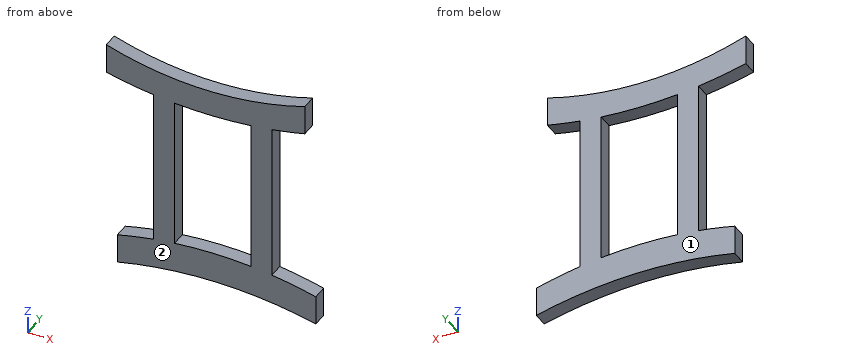
from build123d import *

# Parameters (mm, degrees)
F1_DEPTH = 6.604


with BuildPart() as f1:
    # F0 (on Front) → F1 (new body)
    with BuildSketch(Plane.XZ):
        with BuildLine():
            ThreePointArc((-43.79801, -38.727241), (-0.659432, -34.440726), (42.30799, -40.195004))
            Line((42.30799, -40.195004), (42.30799, -27.495004))
            ThreePointArc((42.30799, -27.495004), (32.83759, -25.203711), (23.254529, -23.442051))
            Line((23.254529, -23.442051), (23.254529, 44.543938))
            ThreePointArc((23.254529, 44.543938), (30.416051, 45.697065), (37.527271, 47.128027))
            Line((37.527271, 47.128027), (37.527271, 59.828027))
            ThreePointArc((37.527271, 59.828027), (-5.639596, 53.881838), (-48.578729, 61.295779))
            Line((-48.578729, 61.295779), (-48.578729, 48.430497))
            ThreePointArc((-48.578729, 48.430497), (-38.380513, 46.14736), (-28.070346, 44.439504))
            Line((-28.070346, 44.439504), (-28.070339, -23.076924))
            ThreePointArc((-28.070339, -23.076924), (-35.967851, -24.372561), (-43.79801, -26.027241))
            Line((-43.79801, -26.027241), (-43.79801, -38.727241))
        make_face()
        with BuildLine():
            Line((-18.977908, -22.038799), (-18.977908, 43.420898))
            ThreePointArc((-18.977908, 43.420898), (-2.406415, 42.716282), (14.162091, 43.487954))
            Line((14.162091, 43.487954), (14.162091, -22.273066))
            ThreePointArc((14.162091, -22.273066), (-2.402361, -21.371167), (-18.977908, -22.038799))
        make_face(mode=Mode.SUBTRACT)
    extrude(amount=F1_DEPTH)


solid = f1.part
Source: CAD feature listing. Evaluate the final solid. Frame: model axes, mm. Face numbers are marked on the shaded views. Round coordinates to 2 decimals unless told otherwise and drop trailing zeros. Order: outer loops, then holes, each group sorted by start corner. A loop starts at its lowest first (then second) coordinate and runs counter-clockwise, first axis right, second up. Notation, with made-up numbers: (55, 83.25) - (63, 83.25) arc R14 ccw to (63, 110.25) - close; hole circle Ø2 at (58.5, -2.5). An arc over 180 degrees is marked (long way). Use a Markdown table: item, result. Add a question column.
1. Section query C-C (y = -4.25). Return the cut outline in (x, z) (1 decimal).
2. Section query A-A (z = 12). Return the cut outline in (x, y), then the cut area to 3 significant figures.
3. Line query: probe 1 along X at (y, z) = (-2.25, 18); probe 2 along Z at (x, y) = (-1, -5.5); probe 3 along Z at (x, y) = (-32, -5.25). Output: solid intervals per line, ascending.
4. Mould query, pull axis Y, two halves, no side actions, for the marked faces 1 and 2. Classes: +Y half, -Y half, draft (parallel to the pull), parting line (faces both ways), or undercut.
5. First-contact query: pin 1 (3.5 mm diameter, centred on y = -4, z = 18.5, fed in from +X); pin 2 (2 mm diameter, centred on x = -7, y = -4, fed in from +Z); pin 3 (1.5 mm diameter, centred on y = -5, z = 2.5, fed in from -X). Flat tips, straight axial feed; report the tip coordinate or a pass-through.
6. Section query D-D (z = -29.5). Return the cut outline in (x, y), then the cut area to 3 significant figures.
7. Section query B-B (x = 36). Return the cut outline in (y, z).
Derived:
| question | item | result |
|---|---|---|
| 1 | outline | (-48.6, 48.4) arc R186.4 ccw to (-28.1, 44.4) - (-28.1, -23.1) arc R175.3 ccw to (-43.8, -26) - (-43.8, -38.7) arc R187.1 cw to (42.3, -40.2) - (42.3, -27.5) arc R175.3 ccw to (23.3, -23.4) - (23.3, 44.5) arc R186.4 ccw to (37.5, 47.1) - (37.5, 59.8) arc R142.1 cw to (-48.6, 61.3) - close; hole (-19, -22) arc R175.3 cw to (14.2, -22.3) - (14.2, 43.5) arc R186.4 cw to (-19, 43.4) - close |
| 2 | outline | (-28.07, -6.6) - (-18.98, -6.6) - (-18.98, 0) - (-28.07, 0) - close; (14.16, -6.6) - (23.25, -6.6) - (23.25, 0) - (14.16, 0) - close |
| 2 | area | 120 mm2 |
| 3 | probe 1 | -28.07 to -18.98, 14.16 to 23.25 |
| 3 | probe 2 | -34.44 to -21.39, 42.72 to 53.88 |
| 3 | probe 3 | -36.54 to -23.68, 45.02 to 56.81 |
| 4 | face 1 | +Y half |
| 4 | face 2 | -Y half |
| 5 | pin 1 | x = 23.25 |
| 5 | pin 2 | z = 53.94 |
| 5 | pin 3 | x = -28.07 |
| 6 | outline | (-43.8, -6.6) - (42.31, -6.6) - (42.31, 0) - (-43.8, 0) - close |
| 6 | area | 569 mm2 |
| 7 | outline | (-6.6, -38.71) - (0, -38.71) - (0, -25.91) - (-6.6, -25.91) - close; (-6.6, 46.8) - (0, 46.8) - (0, 59.38) - (-6.6, 59.38) - close |
